Read the model definition and answer for the solid it produces. Units are mm, in the model's axes. Round coordinates to 2 decimals unless told otherwise and drop trailing zeros. Loops run counter-clockwise (first coordinate to the right, second up) from the corner with the lowest first, then second, coordinate; pieces in that order, holes last. Notation, with made-up numbers: M 57,74.25 L 70,74.25 A29 ccw 70,106.25 Z; hole C 27.25,72.25 d5. An arc over 180 degrees is marked long. Answer as CSV lines item,"result".
```python
from build123d import *

# Parameters (mm, degrees)
BOSS_EXTRUDE1_DEPTH = 3
SKETCH2_R           = 2.5
BOSS_EXTRUDE2_DEPTH = 34
BOSS_EXTRUDE3_DEPTH = 3
SKETCH4_R           = 1.5
CUT_EXTRUDE1_DEPTH  = 41
CHAMFER1_SIZE       = 0.5


with BuildPart() as part:
    # Sketch1 → Boss-Extrude1 (new body)
    with BuildSketch(Plane(origin=(0, 0, 0), x_dir=(1, 0, 0), z_dir=(0, 1, 0))):
        Polygon((1.5, -2.598076211), (3, 0), (1.5, 2.598076211), (-1.5, 2.598076211), (-3, 0), (-1.5, -2.598076211), align=None)
    extrude(amount=BOSS_EXTRUDE1_DEPTH)

    # Sketch2 → Boss-Extrude2 (add)
    with BuildSketch(Plane(origin=(0, 3, 0), x_dir=(1, 0, 0), z_dir=(0, 1, 0))):
        Circle(SKETCH2_R)
    extrude(amount=BOSS_EXTRUDE2_DEPTH)

    # Sketch3 → Boss-Extrude3 (add)
    with BuildSketch(Plane(origin=(0, 37, 0), x_dir=(1, 0, 0), z_dir=(0, 1, 0))):
        Polygon((1.5, -2.598076211), (3, 0), (1.5, 2.598076211), (-1.5, 2.598076211), (-3, 0), (-1.5, -2.598076211), align=None)
    extrude(amount=BOSS_EXTRUDE3_DEPTH)

    # Sketch4 → Cut-Extrude1 (cut, through all)
    with BuildSketch(Plane(origin=(0, 40, 0), x_dir=(1, 0, 0), z_dir=(0, 1, 0))):
        Circle(SKETCH4_R)
    extrude(amount=-CUT_EXTRUDE1_DEPTH, mode=Mode.SUBTRACT)

    # Chamfer1
    chamfer1_edges = [part.edges().sort_by_distance(p)[0] for p in [
        (-1.5, 0, 0),
        (-1.5, 40, 0),
    ]]
    chamfer(chamfer1_edges, length=CHAMFER1_SIZE)


solid = part.part
```
1) Find section B-B, the plane y = 8.5. Give the vertices of the cut face in (x, z), then the cut area to 3 significant figures.
Evaluation:
outline,"C 0,0 d5; hole C 0,0 d3"
area,"12.6 mm^2"
2) Each of these flat-tipped pins is pushed along its axis until it touches: P1, Ø1.5, axis at x = 1, y = 22.5, coming from the -Z side; P2, Ø3, axis at x = -2.5, y = 15.5, coming from the -Z side; P3, Ø1.6, axis at x = 0.5, z = 1, coming from the +Y side. Where does it stop, or does it pass through?
Evaluation:
P1,"stops at z = -2.49"
P2,"stops at z = -2.29"
P3,"stops at y = 39.92"
3) Determine the mould class of faces 1 (the flat face through (0, 38, 2.598)), 2 (the cylindrical face through (-0.54, 19.76, 2.44)), 3 (the cylindrical face through (-1.5, 20.27, -0.07)) for opening direction X: released by +X, released by -X, zero draft, split by the parting line, or undercut.
Evaluation:
face 1,"zero draft"
face 2,"split by the parting line"
face 3,"undercut"
4) Find section A-A, the plane x = 0. Give the vertices of the cut face in (y, z), then the cut area to 3 significant figures.
Evaluation:
outline,"M 0,-2.6 L 3,-2.6 L 3,-2.5 L 37,-2.5 L 37,-2.6 L 40,-2.6 L 40,-2 L 39.5,-1.5 L 0.5,-1.5 L 0,-2 Z; M 0,2 L 0.5,1.5 L 39.5,1.5 L 40,2 L 40,2.6 L 37,2.6 L 37,2.5 L 3,2.5 L 3,2.6 L 0,2.6 Z"
area,"80.7 mm^2"
5) Straight lines are drawn through the part: line 1 (Z direction, x = 0, y = 17); line 2 (Z direction, x = -0.5, y = 14). For each, find the intervals that lie inside material, in ascending order.
Evaluation:
line 1,"z = -2.5 to -1.5, 1.5 to 2.5"
line 2,"z = -2.45 to -1.41, 1.41 to 2.45"
